from build123d import *

# Parameters (mm, degrees)
F0_W     = 400.05
F0_H     = 584.2
F1_DEPTH = 3.175
F3_DEPTH = 25.4


with BuildPart() as f1:
    # F0 (on Top) → F1 (new body)
    with BuildSketch(Plane.XY):
        Rectangle(F0_W, F0_H)
    extrude(amount=F1_DEPTH)

    # F2 (on face) → F3 (join)
    with BuildSketch(Plane.XZ.offset(292.1)):
        with BuildLine():
            ThreePointArc((-200.025, 3.175), (-202.2700640303, -2.2450640303), (-196.85, 0))
            Line((-196.85, 0), (-200.025, 0))
            Line((-200.025, 0), (-200.025, 3.175))
        make_face()
    extrude(amount=-F3_DEPTH)

    # F4: F1 across plane


with BuildPart() as f1_1:
    add(f1.part)
    add(f1.part.mirror(Plane.XZ))


solid = f1_1.part
For this review, take the finished solid that the model builds, in its own axes (mm). Coordinates: 2 decimals unless noted, no trailing zeros. Order: outer loops, then holes, each group sorted by start corner. A loop starts at its lowest first (then second) coordinate and runs counter-clockwise, first axis right, second up. Notation, with made-up numbers: (87.25, 76.5) -> (131.25, 76.5) arc R16 cw to (131.25, 96.5) -> close; hole circle Ø2 at (-8.75, 25). An arc over 180 degrees is marked (long way). Return JSON: item names as keys, results as strings.
1. We need section A-A on y = 224.5. Write out the cut boundary in (x, z) (3 decimals), and give its area (3 significant figures).
Answer block:
{"outline": "(-200.025, 0) -> (200.025, 0) -> (200.025, 3.175) -> (-200.025, 3.175) -> close", "area": "1,270 mm²"}
2. For line 1 (Z direction, x = 62, y = -210) (3 decimals); line 2 (X direction, y = -114, z = 1) (3 decimals), list the stretches that pass through material, from the lowest coordinate up. Write a range as from..to.
Answer block:
{"line 1": "0..3.175", "line 2": "-200.025..200.025"}
3. We need section B-B on x = 33. Write out the cut boundary in (y, z) (3 decimals), and give its area (3 significant figures).
Answer block:
{"outline": "(-292.1, 0) -> (292.1, 0) -> (292.1, 3.175) -> (-292.1, 3.175) -> close", "area": "1,850 mm²"}
4. For pin 1 Ø12 at (x, y) = (-115, 113) entering from -Z; pin 2 Ø3.5 at (y, z) = (-7.5, 1.5) entering from -X (3 decimals), all flat-tipped, find the tip position at first contact; note any pin that passes through.
Answer block:
{"pin 1": "z = 0", "pin 2": "x = -200.025"}
